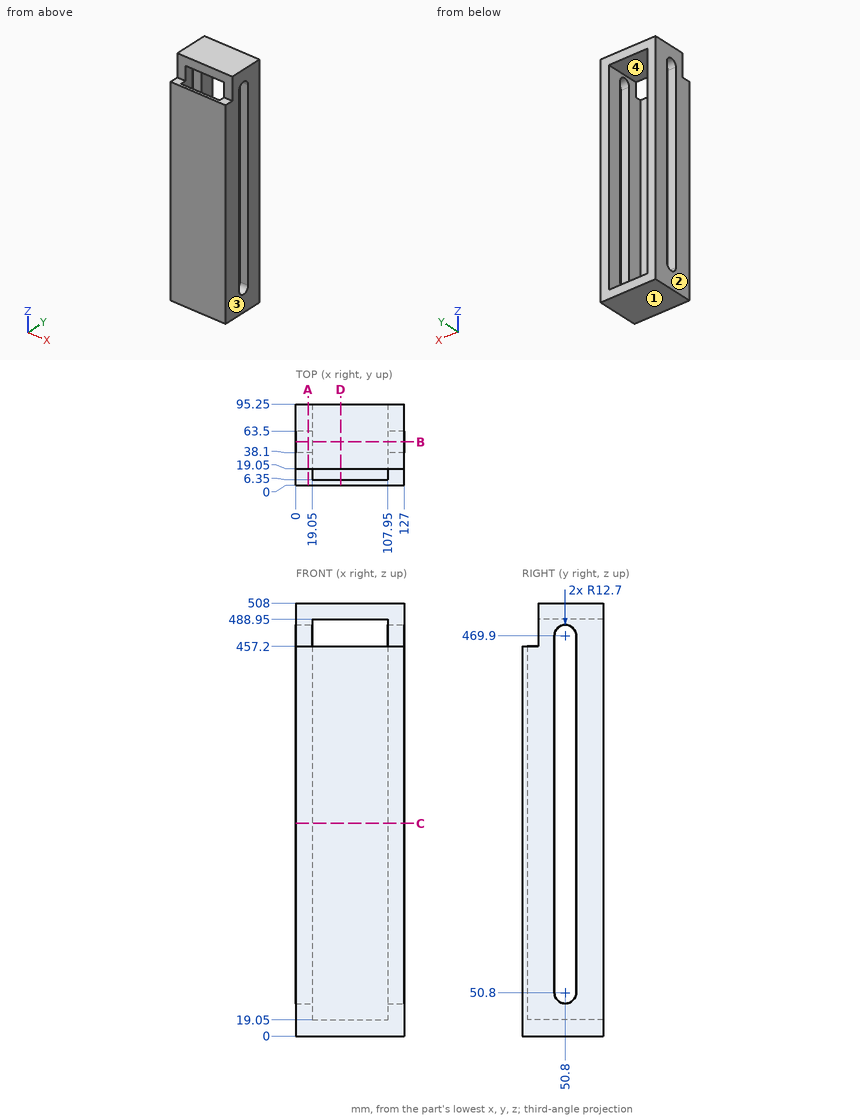
Could you check a few things on this drawing? It's one solid part, dimensions in mm from its lowest x, y, z. Give positions to 0.01 mm unless a question says otherwise; leave off trailing zeros. Order: outer loops, then holes, each group sorted by start corner. A loop starts at its lowest first (then second) coordinate and runs counter-clockwise, first axis right, second up. Notation, with made-up numbers: (30.25, 52.25) - (43.25, 52.25) arc R26 ccw to (43.25, 67.25) - close; hole circle Ø10 at (55.25, 7.25). An arc over 180 degrees is marked (long way). Answer as a JSON object with one key per item and string values. Group by question number.
Item 1: For P1, Ø5.5, axis at x = 39, y = 6, coming from the +Z side, with a flat end and sliding along its axis, tell me the tip position at first contact or that it passes through.
Item 2: If we mould it in two halves opening along X, with no side actions, what happens to the marked faces 1, 2, 3 and 4? For each: pulls with the +X half, pulls with the -X half, needs draft (parallel to the pull), parting line crosses it, or undercut.
Item 3: If we section it at C-C on z = 249.5: Please give me the cut outline in (x, y), and give its area (3 significant figures).
Item 4: Please list where these lines run through material, in increasing order: probe 1 along Z at (x, y) = (101.5, 19.5); probe 2 along X at (y, z) = (24.5, 120); probe 3 along Y at (x, z) = (18, 157).
Item 5: If we section it at D-D on x = 52.5: Please give me the cut outline in (y, z).
Item 6: If we section it at A-A on x = 14.5: Please give me the cut outline in (y, z), and give its area (3 significant figures).
Item 7: If we section it at B-B on y = 50.8: Please give me the cut outline in (x, z), and give its area (3 significant figures).
Result set:
{
 "1": {"P1": "z = 457.2"},
 "2": {"face 1": "needs draft", "face 2": "pulls with the -X half", "face 3": "pulls with the +X half", "face 4": "undercut"},
 "3": {"outline": "(0, 0) - (127, 0) - (127, 38.1) - (107.95, 38.1) - (107.95, 6.35) - (19.05, 6.35) - (19.05, 38.1) - (0, 38.1) - close; (0, 63.5) - (19.05, 63.5) - (19.05, 95.25) - (0, 95.25) - close; (107.95, 63.5) - (127, 63.5) - (127, 95.25) - (107.95, 95.25) - close", "area": "3,230 mm²"},
 "4": {"probe 1": "0 to 19.05, 488.95 to 508", "probe 2": "0 to 19.05, 107.95 to 127", "probe 3": "0 to 38.1, 63.5 to 95.25"},
 "5": {"outline": "(0, 0) - (95.25, 0) - (95.25, 19.05) - (6.35, 19.05) - (6.35, 457.2) - (0, 457.2) - close; (19.05, 488.95) - (95.25, 488.95) - (95.25, 508) - (19.05, 508) - close"},
 "6": {"outline": "(0, 0) - (95.25, 0) - (95.25, 508) - (19.05, 508) - (19.05, 457.2) - (0, 457.2) - close; hole (38.1, 50.8) arc R12.7 ccw to (63.5, 50.8) - (63.5, 469.9) arc R12.7 ccw to (38.1, 469.9) - close", "area": "36,300 mm²"},
 "7": {"outline": "(0, 0) - (127, 0) - (127, 38.1) - (107.95, 38.1) - (107.95, 19.05) - (19.05, 19.05) - (19.05, 38.1) - (0, 38.1) - close; (0, 482.6) - (19.05, 482.6) - (19.05, 488.95) - (107.95, 488.95) - (107.95, 482.6) - (127, 482.6) - (127, 508) - (0, 508) - close", "area": "5,810 mm²"}
}
